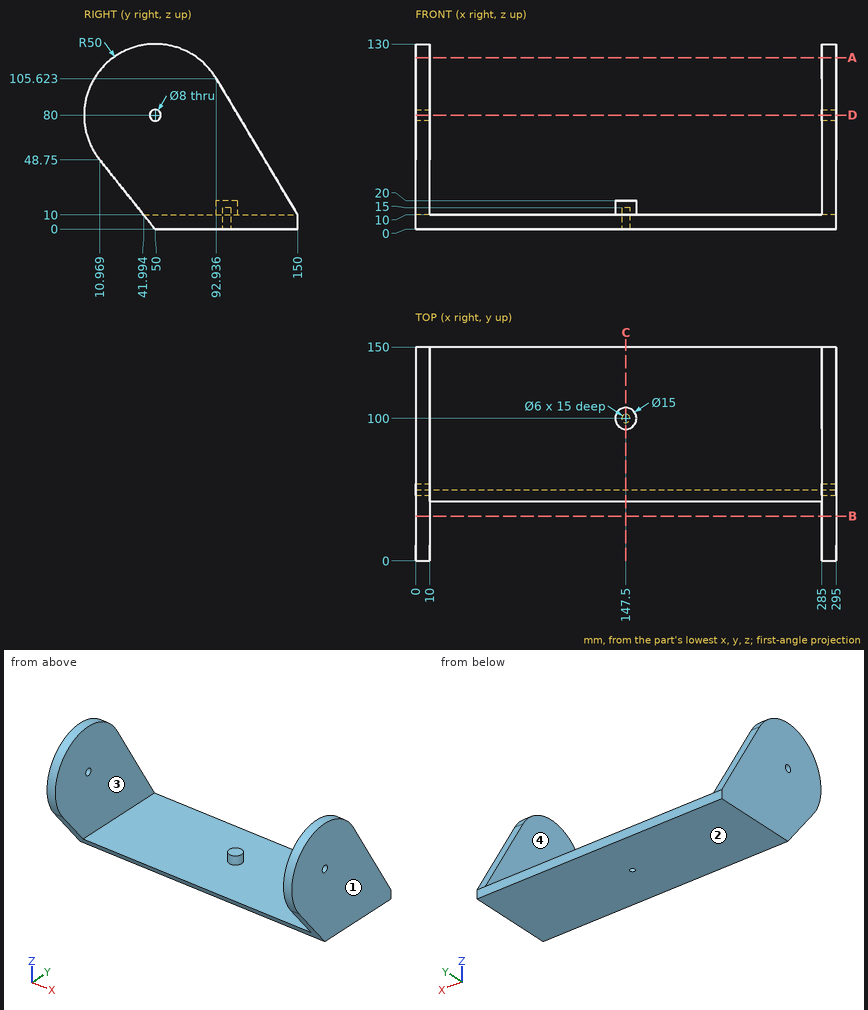
Could you check a few things on this drawing? It's one solid part, dimensions in mm from its lowest x, y, z. Give positions to 0.01 mm unless a question says otherwise; leave off trailing zeros. Order: outer loops, then holes, each group sorted by start corner. A loop starts at its lowest first (then second) coordinate and runs counter-clockwise, first axis right, second up. Notation, with made-up numbers: (89, 72.5) - (113, 72.5) arc R24 cw to (113, 108.5) - close; hole circle Ø6 at (15.25, -18). An arc over 180 degrees is marked (long way). One line per question, with ' | ' between items. Start each with the question number.
Item 1: I'm going to push flat-ended pins straight in: pin 1 Ø5.5 at (x, y) = (147.5, 100) entering from +Z; pin 2 Ø2 at (x, y) = (71, 46.5) entering from +Z. Where does each tip first touch, or does it pass through?
Item 2: Thinking about a two-plate mould opening in X: for the marked faces 1, 2, 3 and 4, which applies, pulls with the +X half, pulls with the -X half, needs draft (parallel to the pull), parting line crosses it, or undercut?
Item 3: I want a section at A-A on z = 120.5. Write out the boundary of the cut face in (x, y).
Item 4: I want a section at D-D on z = 80. Write out the boundary of the cut face in (x, y).
Item 5: I want a section at B-B on y = 31.5. Write out the boundary of the cut face in (x, z).
Item 6: I want a section at C-C on x = 147.5. Write out the boundary of the cut face in (y, z), then the cut area to 3 significant figures.
Item 7: I need wall thicknesses on probe 1 along X at (y, z) = (103.5, 26); probe 2 along X at (y, z) = (98, 15.5); probe 3 along Z at (x, y) = (252, 143). Which ranges of each line are inside material? Lowest first, please. Write a range as [from, to].
Verdict:
1) pin 1: z = 20 | pin 2: z = 10
2) face 1: pulls with the +X half | face 2: needs draft | face 3: undercut | face 4: undercut
3) outline: (0, 20.68) - (10, 20.68) - (10, 79.32) - (0, 79.32) - close; (285, 20.68) - (295, 20.68) - (295, 79.32) - (285, 79.32) - close
4) outline: (0, 0) - (10, 0) - (10, 46) - (0, 46) - close; (0, 54) - (10, 54) - (10, 108.23) - (0, 108.23) - close; (285, 0) - (295, 0) - (295, 46) - (285, 46) - close; (285, 54) - (295, 54) - (295, 108.23) - (285, 108.23) - close
5) outline: (0, 23.11) - (10, 23.11) - (10, 126.45) - (0, 126.45) - close; (285, 23.11) - (295, 23.11) - (295, 126.45) - (285, 126.45) - close
6) outline: (41.99, 10) - (50, 0) - (97, 0) - (97, 15) - (103, 15) - (103, 0) - (150, 0) - (150, 10) - (107.5, 10) - (107.5, 20) - (92.5, 20) - (92.5, 10) - close | area: 1,100 mm^2
7) probe 1: [0, 10], [285, 295] | probe 2: [0, 10], [140.27, 154.73], [285, 295] | probe 3: [0, 10]
